```python
from build123d import *

# Parameters (mm, degrees)
ESQUISSE1_W             = 45
ESQUISSE1_H             = 15
BOSS_EXTRU_1_DEPTH      = 4
CONG_1_R                = 5
CONG_2_R                = 3
ESQUISSE2_R             = 1.5
ENL_V_MAT_EXTRU_1_DEPTH = 5


with BuildPart() as part:
    # Esquisse1 → Boss.-Extru.1 (new body)
    with BuildSketch(Plane.XY):
        Rectangle(ESQUISSE1_W, ESQUISSE1_H)
    extrude(amount=BOSS_EXTRU_1_DEPTH)

    # Congé1
    cong_1_edges = [part.edges().sort_by_distance(p)[0] for p in [
        (-22.5, 7.5, 2),
        (22.5, 7.5, 2),
        (22.5, -7.5, 2),
        (-22.5, -7.5, 2),
    ]]
    fillet(cong_1_edges, radius=CONG_1_R)

    # Congé2
    cong_2_edges = [part.edges().sort_by_distance(p)[0] for p in [
        (22.5, 0, 4),
        (0, -7.5, 4),
        (-22.5, 0, 4),
        (0, 7.5, 4),
        (21.035533906, 6.035533906, 4),
        (-21.035533906, 6.035533906, 4),
        (-21.035533906, -6.035533906, 4),
        (21.035533906, -6.035533906, 4),
    ]]
    fillet(cong_2_edges, radius=CONG_2_R)

    # Esquisse2 → Enlèv. mat.-Extru.1 (cut, through all)
    with BuildSketch(Plane.XY.offset(4)):
        with Locations((-12.5, 1.5)):
            Circle(ESQUISSE2_R)
        with Locations((12.5, 1.5)):
            Circle(ESQUISSE2_R)
    extrude(amount=-ENL_V_MAT_EXTRU_1_DEPTH, mode=Mode.SUBTRACT)


solid = part.part
```
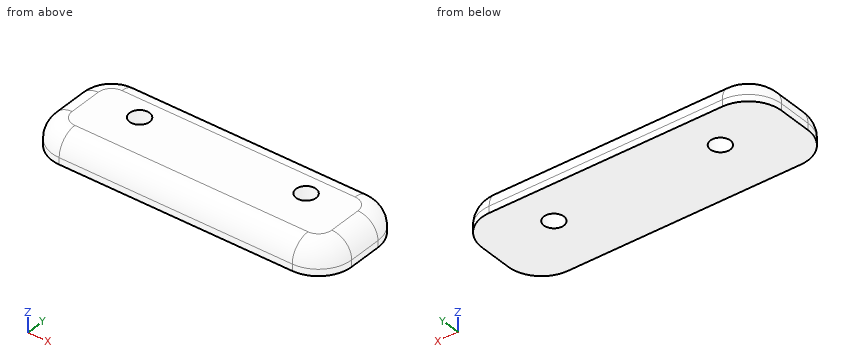
Geometry: final body of the model. Coordinates: model frame, mm. Round coordinates to 2 decimals unless told otherwise and drop trailing zeros. Write each loop counter-clockwise with the first axis right and the second up, starting at its lowest first coordinate (ties: lowest second). Pieces come first, ordered by that corner, then holes.
Item 1: Pin query (flat end, axial travel): P1, Ø2.5, axis at x = -12.5, y = 1.5, coming from the -Z side; P2, Ø2, axis at y = -5, z = 0.5, coming from the -X side; P3, Ø1.5, axis at y = 5.5, z = 1, coming from the -X side. Return the tip coordinate at first contact, or that it passes through.
Item 2: Material intervals for L1, parallel to Y at x = 12.5, z = 0.9; L2, parallel to Y at x = -12.5, z = 3; L3, parallel to X at y = 6, z = 2.95, sorted ascending.
Item 3: Section query B-B (x = 12.5). Return loops of the section in (y, z), plus the area to 3 significant figures.
Item 4: Section query A-A (y = 1.5). Return loops of the section in (x, z).
Item 5: Section query C-C (x = 2.5). Return loops of the section in (y, z), plus the area to 3 significant figures.
Item 6: Section query D-D (z = 2.85). Give the number of separate pieces and of enclosed holes in the cut face, plus the area to 3 significant figures.
Completed:
1. P1: passes through
1. P2: stops at x = -22.27
1. P3: stops at x = -21.97
2. L1: y = -7.5 to 0, 3 to 7.5
2. L2: y = -6.74 to 0, 3 to 6.74
2. L3: x = -19.96 to 19.96
3. outline: (-7.5, 0) - (0, 0) - (0, 4) - (-4.5, 4) arc R3 ccw to (-7.5, 1) - close; (3, 0) - (7.5, 0) - (7.5, 1) arc R3 ccw to (4.5, 4) - (3, 4) - close
3. area: 44.1 mm2
4. outline: (-22.5, 0) - (-14, 0) - (-14, 4) - (-19.5, 4) arc R3 ccw to (-22.5, 1) - close; (-11, 0) - (11, 0) - (11, 4) - (-11, 4) - close; (14, 0) - (22.5, 0) - (22.5, 1) arc R3 ccw to (19.5, 4) - (14, 4) - close
5. outline: (-7.5, 0) - (7.5, 0) - (7.5, 1) arc R3 ccw to (4.5, 4) - (-4.5, 4) arc R3 ccw to (-7.5, 1) - close
5. area: 56.1 mm2
6. separate pieces: 1
6. enclosed holes: 2
6. area: 570 mm2
